Geometry check sheet. Reference: drawing and pictorial views, mm from the part's lowest x, y, z. A direction names the side the tool comes from. Round coordinates to 2 decimals unless told otherwise and drop trailing zeros. Write each loop counter-clockwise with the first axis right and the second up, starting at its lowest first coordinate (ties: lowest second). Pieces come first, ordered by that corner, then holes.
Item 1: Section check B-B, the plane z = 14.5. Record the cut outline in (x, y), plus the area to 3 significant figures.
Item 2: Material ranges on line 1 along X through (y, z) = (15.5, 21.5); line 2 along Y through (x, z) = (28.5, 28), recorded low to high.
Item 3: Release check for a two-part mould opening along X. For the marked faces 1, 2, 3 and 4 record: pulls with the +X half, pulls with the -X half, needs draft (parallel to the pull), parting line crosses it, or undercut.
Item 4: Section check D-D, the plane y = 51. Record the cut outline in (x, z).
Item 5: Section check C-C, the plane x = 32.5. Record the cut outline in (y, z).
Item 6: Section check A-A, the plane y = 41. Record the cut outline in (x, z), plus the area to 3 significant figures.
Item 7: Set-up check for the marked faces 5 and 6: record each of +Z, -Z, +X, -X, +Y, -Y from which the full face is reachable in a straight line by a thin tool's end or side.
Item 8: Depth check by flat-ended pin: pin 1 (10 mm diameter, centred on x = 7, y = 30.5, fed in from +Z); pin 2 (18.5 mm diameter, centred on x = 13, z = 10.5, fed in from -Y). Enter the tip coordinate at first touch or a pass-through.
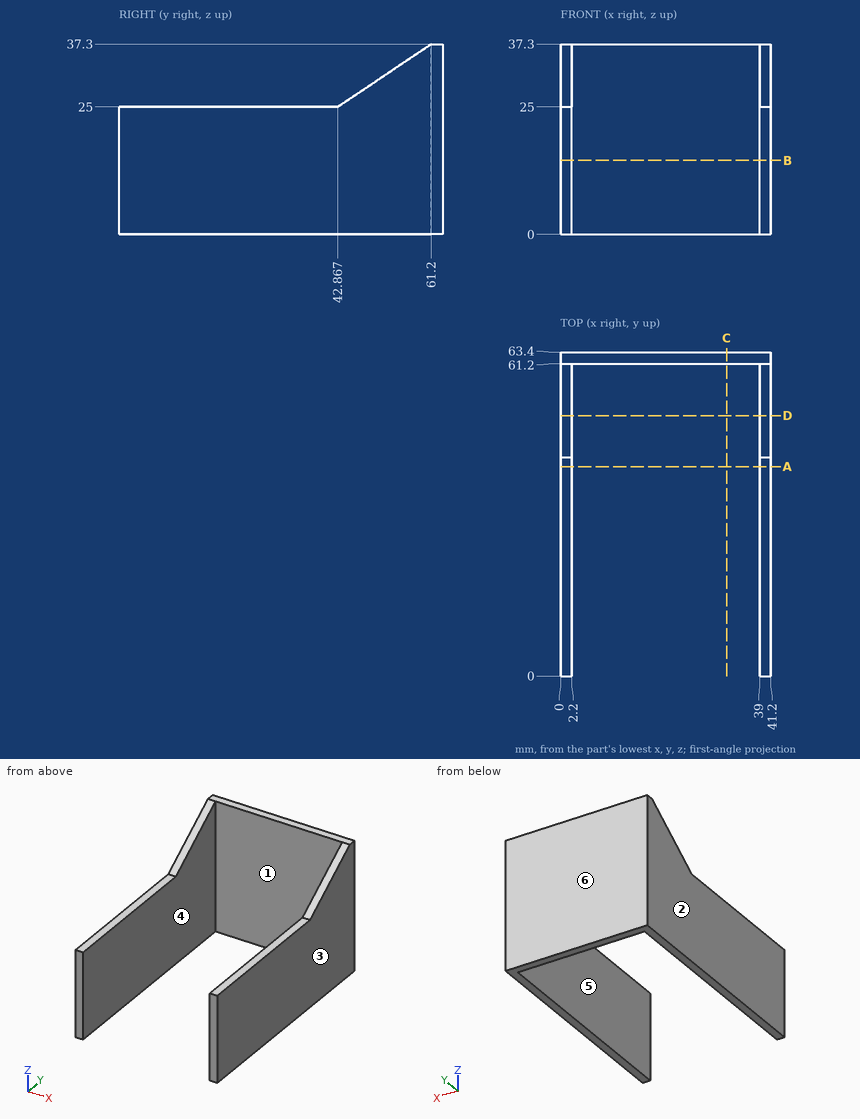
Values found:
1. outline: (0, 0) - (2.2, 0) - (2.2, 61.2) - (39, 61.2) - (39, 0) - (41.2, 0) - (41.2, 63.4) - (0, 63.4) - close
1. area: 360 mm2
2. line 1: x = 0 to 2.2, 39 to 41.2
2. line 2: y = 61.2 to 63.4
3. face 1: undercut
3. face 2: pulls with the -X half
3. face 3: pulls with the +X half
3. face 4: undercut
4. outline: (0, 0) - (2.2, 0) - (2.2, 30.46) - (0, 30.46) - close; (39, 0) - (41.2, 0) - (41.2, 30.46) - (39, 30.46) - close
5. outline: (61.2, 0) - (63.4, 0) - (63.4, 37.3) - (61.2, 37.3) - close
6. outline: (0, 0) - (2.2, 0) - (2.2, 25) - (0, 25) - close; (39, 0) - (41.2, 0) - (41.2, 25) - (39, 25) - close
6. area: 110 mm2
7. face 5: +Z, -Z, -Y
7. face 6: +Z, -Z, +X, -X, +Y
8. pin 1: stops at z = 25
8. pin 2: stops at y = 61.2
